from build123d import *

# Parameters (mm, degrees)
Y_KSEKLIK_EKSTR_ZYON1_DEPTH      = 39.25
Y_KSEKLIK_EKSTR_ZYON1_DEPTH_BACK = 39.25
IZIM1_R                          = 6
IZIM1_R_2                        = 4.1
IZIM2_R                          = 7
IZIM2_R_2                        = 4.1
Y_KSEKLIK_EKSTR_ZYON2_DEPTH      = 10
RADYUS1_R                        = 10


with BuildPart() as part:
    # Çizim1 → Yükseklik-Ekstrüzyon1 (new, two sides: drawn at the far end of the back side and taken through both)
    with BuildSketch(Plane(origin=(0, 0, 0), x_dir=(1, 0, 0), z_dir=(0, 1, 0)).offset(-Y_KSEKLIK_EKSTR_ZYON1_DEPTH_BACK)):
        with Locations(Location((0, 0, 0), (0, 0, 270))):
            Circle(IZIM1_R)
        with Locations(Location((0, 0, 0), (0, 0, 270))):
            Circle(IZIM1_R_2, mode=Mode.SUBTRACT)
    extrude(amount=Y_KSEKLIK_EKSTR_ZYON1_DEPTH + Y_KSEKLIK_EKSTR_ZYON1_DEPTH_BACK)

    # Çizim2 → Yükseklik-Ekstrüzyon2 (add)
    with BuildSketch(Plane(origin=(0, 39.25, 0), x_dir=(1, 0, 0), z_dir=(0, 1, 0))):
        with Locations(Location((0, 0, 0), (0, 0, 270))):
            Circle(IZIM2_R)
        with Locations(Location((0, 0, 0), (0, 0, 270))):
            Circle(IZIM2_R_2, mode=Mode.SUBTRACT)
    y_kseklik_ekstr_zyon2 = extrude(amount=-Y_KSEKLIK_EKSTR_ZYON2_DEPTH)

    # Aynalama1: Yükseklik-Ekstrüzyon2 across plane
    add(y_kseklik_ekstr_zyon2.mirror(Plane.ZX))

    # Radyus1
    # the kernel refuses this fillet: 10 mm, written as the material it adds along each edge
    with BuildSketch(Plane(origin=(0, 29.25, 0), x_dir=(0, 0, 1), z_dir=(1, 0, 0))) as radyus1_piece_1:
        with BuildLine():
            CenterArc((16, 4.358898944), RADYUS1_R, 180, 25.841932763)
            Line((7, 0), (6.82, -0.087177979))
            ThreePointArc((6.82, -0.087177979), (6.5, -0.2), (6, -0.2))
            Line((6, -0.2), (5.8, 0))
            Line((5.8, 0), (5.8, 4.358898944))
            Line((5.8, 4.358898944), (6, 4.358898944))
        make_face()
    revolve(axis=Axis((0, 29.25, 0), (0, -1, 0)))
    with BuildSketch(Plane(origin=(0, -29.25, 0), x_dir=(0, 0, 1), z_dir=(-1, 0, 0))) as radyus1_piece_2:
        with BuildLine():
            CenterArc((16, 4.358898944), RADYUS1_R, 180, 25.841932763)
            Line((7, 0), (6.82, -0.087177979))
            ThreePointArc((6.82, -0.087177979), (6.5, -0.2), (6, -0.2))
            Line((6, -0.2), (5.8, 0))
            Line((5.8, 0), (5.8, 4.358898944))
            Line((5.8, 4.358898944), (6, 4.358898944))
        make_face()
    revolve(axis=Axis((0, -29.25, 0), (0, 1, 0)))


solid = part.part
Model file for the job. Use its own axes, mm. Round coordinates to 2 decimals unless told otherwise and drop trailing zeros. Loops run counter-clockwise (first coordinate to the right, second up) from the corner with the lowest first, then second, coordinate; pieces in that order, holes last. Notation, with made-up numbers: (-14, 30.5) - (8, 30.5) arc R17 cw to (8, 40.5) - close; hole circle Ø3 at (58, 55.25). An arc over 180 degrees is marked (long way). Write each question's results on one line, items separated by ' | '.
(1) Pin check, flat tips, straight feed: pin 1 (6 mm diameter, centred on x = 1.5, y = 18, fed in from +Z); pin 2 (3 mm diameter, centred on y = -27, z = -3, fed in from +X); pin 3 (6 mm diameter, centred on y = 14.5, z = 2.5, fed in from -X). Stop position of each tip, or through.
Answer below:
pin 1: stops at z = 6 | pin 2: stops at x = 6.22 | pin 3: stops at x = -6
(2) Saw through at A-A, the plane z = 0. List the corners of the cut face in (x, y), then the cut area to 3 significant figures.
Answer below:
outline: (-7, -39.25) - (-4.1, -39.25) - (-4.1, 39.25) - (-7, 39.25) - (-7, 29.25) arc R10 cw to (-6, 24.89) - (-6, -24.89) arc R10 cw to (-7, -29.25) - close; (4.1, -39.25) - (7, -39.25) - (7, -29.25) arc R10 cw to (6, -24.89) - (6, 24.89) arc R10 cw to (7, 29.25) - (7, 39.25) - (4.1, 39.25) - close | area: 344 mm^2
(3) Saw through at C-C, the plane y = 32.5. List the corners of the cut face in (x, z), then the cut area to 3 significant figures.
Answer below:
outline: circle Ø14 at (0, 0); hole circle Ø8.2 at (0, 0) | area: 101 mm^2
(4) Saw through at B-B, the plane x = 0. List the corners of the cut face in (y, z), then the cut area to 3 significant figures.
Answer below:
outline: (-39.25, -7) - (-29.25, -7) arc R10 cw to (-24.89, -6) - (24.89, -6) arc R10 cw to (29.25, -7) - (39.25, -7) - (39.25, -4.1) - (-39.25, -4.1) - close; (-39.25, 4.1) - (39.25, 4.1) - (39.25, 7) - (29.25, 7) arc R10 cw to (24.89, 6) - (-24.89, 6) arc R10 cw to (-29.25, 7) - (-39.25, 7) - close | area: 344 mm^2
(5) Mould opens along Y. For faces 1 (the flat face through (-3.01, -39.25, 3.01)), 2 (the cylindrical face through (1.802, -0.348, 5.723)), 3 (the flat face through (-3.01, 39.25, 3.01)), 4 (the cylindrical face through (-6.834, 34.32, -1.517)) say: released by +Y, released by -Y, zero draft, split by the parting line, or undercut.
Answer below:
face 1: released by -Y | face 2: undercut | face 3: released by +Y | face 4: zero draft
(6) Wall check: L1, parallel to X at y = 22, z = 0; L2, parallel to X at y = 23, z = -2.75; L3, parallel to Z at x = 1.5, y = 11. Give the ranges that are in metal, low to high.
Answer below:
L1: x = -6 to -4.1, 4.1 to 6 | L2: x = -5.33 to -3.04, 3.04 to 5.33 | L3: z = -5.81 to -3.82, 3.82 to 5.81
(7) Saw through at D-D, the plane y = -12. List the corners of the cut face in (x, z).
Answer below:
outline: circle Ø12 at (0, 0); hole circle Ø8.2 at (0, 0)
